Geometry check sheet. Reference: drawing and pictorial views, mm from the part's lowest x, y, z. A direction names the side the tool comes from. Round coordinates to 2 decimals unless told otherwise and drop trailing zeros. Order: outer loops, then holes, each group sorted by start corner. A loop starts at its lowest first (then second) coordinate and runs counter-clockwise, first axis right, second up.
(1) Thickness scan on L1, parallel to Y at x = 3.5, z = 7.4; L2, parallel to X at y = 32, z = 3; L3, parallel to X at y = 24.85, z = 9.05. Record the ranges inside material, lowest first.
(2) Cross-section at C-C on z = 7. Enter the section's corners in (x, y).
(3) Set-up check for the marked faces 5, 6 and 7: record each of +Z, -Z, +X, -X, +Y, -Y from which the full face is reachable in a straight line by a thin tool's end or side.
(4) Cross-section at D-D on x = 11.75. Enter the section's corners in (y, z), and give its area (3 significant figures).
(5) Draft check along X on the marked faces 1, 2, 3 and 4. Enter one of: pulls with the +X half, pulls with the -X half, needs draft (parallel to the pull), parting line crosses it, or undercut.
(6) Cross-section at A-A on z = 2.25. Enter the section's corners in (x, y).
(7) Gauge pin test, flat ends, axial feed: P1, Ø5, axis at x = 10, y = 3, coming from the +Z side; P2, Ø0.9, axis at x = 23.5, y = 25.5, coming from the +Z side. Record the tip position at first contact, or that the pin passes through.
(8) Cross-section at B-B on y = 32. Enter the section's corners in (x, z), and give its area (4 significant figures).
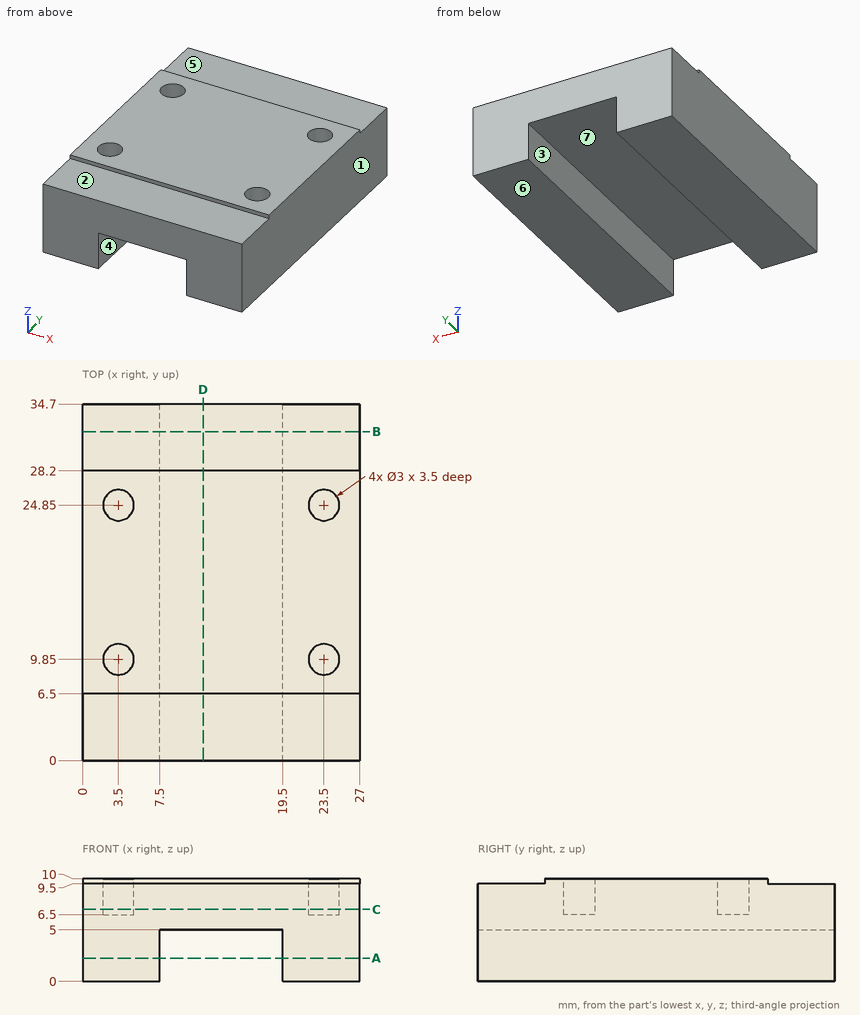
Found:
1. L1: y = 0 to 8.35, 11.35 to 23.35, 26.35 to 34.7
1. L2: x = 0 to 7.5, 19.5 to 27
1. L3: x = 0 to 2, 5 to 22, 25 to 27
2. outline: (0, 0) - (27, 0) - (27, 34.7) - (0, 34.7) - close; hole circle Ø3 at (3.5, 9.85); hole circle Ø3 at (3.5, 24.85); hole circle Ø3 at (23.5, 9.85); hole circle Ø3 at (23.5, 24.85)
3. face 5: +Z, +X, -X, +Y
3. face 6: -Z, +X, -X, +Y, -Y
3. face 7: -Z, +Y, -Y
4. outline: (0, 5) - (34.7, 5) - (34.7, 9.5) - (28.2, 9.5) - (28.2, 10) - (6.5, 10) - (6.5, 9.5) - (0, 9.5) - close
4. area: 167 mm2
5. face 1: pulls with the +X half
5. face 2: needs draft
5. face 3: undercut
5. face 4: undercut
6. outline: (0, 0) - (7.5, 0) - (7.5, 34.7) - (0, 34.7) - close; (19.5, 0) - (27, 0) - (27, 34.7) - (19.5, 34.7) - close
7. P1: stops at z = 9.5
7. P2: stops at z = 6.5
8. outline: (0, 0) - (7.5, 0) - (7.5, 5) - (19.5, 5) - (19.5, 0) - (27, 0) - (27, 9.5) - (0, 9.5) - close
8. area: 196.5 mm2
